Source: CAD feature listing. Evaluate the final solid. Frame: model axes, mm. Coordinates: 2 decimals unless noted, no trailing zeros. Order: outer loops, then holes, each group sorted by start corner. A loop starts at its lowest first (then second) coordinate and runs counter-clockwise, first axis right, second up.
```python
from build123d import *

# Parameters (mm, degrees)
F0_W     = 450
F0_H     = 50
F1_DEPTH = 30
F2_R     = 15
F3_W     = 10
F3_H     = 100
F4_DEPTH = 50.001
F5_R     = 2.5
F7_D     = 10
F7_DEPTH = 100
F8_R     = 10
F9_DEPTH = 30.001


with BuildPart() as f1:
    # F0 (on Right) → F1 (new body)
    with BuildSketch(Plane.YZ):
        with Locations((225, 25)):
            Rectangle(F0_W, F0_H)
    extrude(amount=F1_DEPTH)

    # F2
    f2_edges = [f1.edges().sort_by_distance(p)[0] for p in [
        (15, 0, 50),
        (15, 0, 0),
    ]]
    fillet(f2_edges, radius=F2_R)

    # F3 (on face) → F4 (cut, through all)
    with BuildSketch(Plane.XY.offset(50)):
        with Locations((15, 400)):
            Rectangle(F3_W, F3_H)
    extrude(amount=-F4_DEPTH, mode=Mode.SUBTRACT)

    # F5
    f5_edges = [f1.edges().sort_by_distance(p)[0] for p in [
        (30, 0, 25),
        (30, 4.393398, 45.606602),
        (30, 4.393398, 4.393398),
        (30, 232.5, 50),
        (30, 232.5, 0),
        (30, 450, 25),
        (0, 0, 25),
        (0, 4.393398, 45.606602),
        (0, 4.393398, 4.393398),
        (0, 232.5, 50),
        (0, 232.5, 0),
        (0, 450, 25),
    ]]
    fillet(f5_edges, radius=F5_R)

    # F7
    with Locations(Plane.YZ.offset(30)):
        with Locations((375, 25), (425, 25)):
            Hole(F7_D / 2, depth=F7_DEPTH)

    # F8 (on face) → F9 (cut, through all)
    with BuildSketch(Plane(origin=(0, 0, 0), x_dir=(0, -1, 0), z_dir=(-1, 0, 0))):
        with Locations((-40, 25)):
            Circle(F8_R)
    extrude(amount=-F9_DEPTH, mode=Mode.SUBTRACT)


solid = f1.part
```
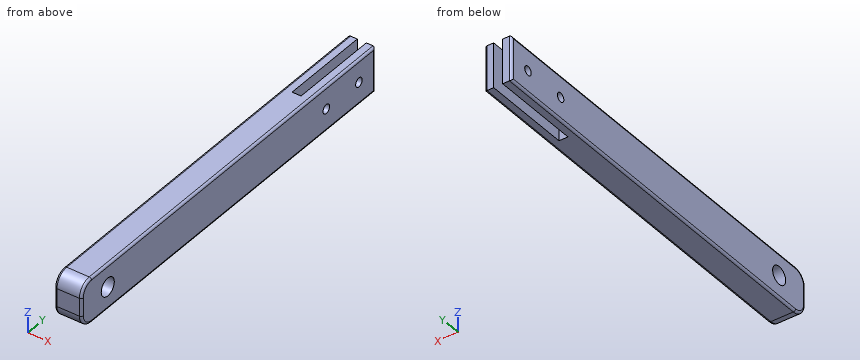
1. Section query C-C on y = 40. Return loops of the section in (x, z).
Findings:
outline: (0, 2.5) arc R2.5 ccw to (2.5, 0) - (27.5, 0) arc R2.5 ccw to (30, 2.5) - (30, 15) - (0, 15) - close; (0, 35) - (30, 35) - (30, 47.5) arc R2.5 ccw to (27.5, 50) - (2.5, 50) arc R2.5 ccw to (0, 47.5) - close
2. Pin query (flat end, axial travel): P1, Ø11, axis at x = 14.5, z = 30, coming from the +Y side; P2, Ø8, axis at y = 425, z = 25, coming from the +X side; P3, Ø4, axis at x = 17, z = 43, coming from the -Y side; P4, Ø1, axis at x = 15, z = 40.5, coming from the +Y side. Return the tip coordinate at first contact, or that it passes through.
Findings:
P1: stops at y = 450
P2: passes through
P3: stops at y = 1.25
P4: stops at y = 350
3. Ray query, line 1 (X direction, y = 369, z = 36.5); line 2 (Z direction, x = 26.5, y = 425); line 3 (Y direction, x = 22.5, z = 27). Return the intervals inside material, ascending.
Findings:
line 1: x = 0 to 10, 20 to 30
line 2: z = 0 to 20, 30 to 50
line 3: y = 0 to 30.2, 49.8 to 370.42, 379.58 to 420.42, 429.58 to 450
4. Section query B-B on z = 25. Count the separate pieces of the cut face and the enclosed holes in it, plus the area to 3 significant figures.
Findings:
separate pieces: 6
enclosed holes: 0
area: 11,500 mm2
5. Section query A-A on y = 393. Return loops of the section in (x, z), plus the area to 3 significant figures.
Findings:
outline: (0, 2.5) arc R2.5 ccw to (2.5, 0) - (10, 0) - (10, 50) - (2.5, 50) arc R2.5 ccw to (0, 47.5) - close; (20, 0) - (27.5, 0) arc R2.5 ccw to (30, 2.5) - (30, 47.5) arc R2.5 ccw to (27.5, 50) - (20, 50) - close
area: 995 mm2
